Could you check a few things on this model? Use its own coordinates, in mm. Face numbers are marked on the shaded views. Coordinates: 2 decimals unless noted, no trailing zeros. Order: outer loops, then holes, each group sorted by start corner. A loop starts at its lowest first (then second) coordinate and runs counter-clockwise, first axis right, second up. Notation, with made-up numbers: (-31, 48) -> (-6, 48) arc R13 ccw to (-6, 62) -> close; hole circle Ø6 at (65.25, 28.5). An arc over 180 degrees is marked (long way). Use a Markdown table: item, result. Add a question column.
1) Thinking about a two-plate mould opening in Y: for the marked faces 1 and 2, which applies, +Y half, -Y half, draft (parallel to the pull), parting line (faces both ways), or undercut?
2) If we section it at A-A (x = -9): Write out the boundary of the cut face in (y, z) (3 decimals), plus the area to 3 significant figures.
3) If we section it at D-D (x = 1): Write out the boundary of the cut face in (y, z), plus the area to 3 significant figures.
4) Will these pins go through, and if not, where does the flat tip stop? pin 1 Ø3.5 at (x, y) = (18, -18.5) entering from -Z; pin 2 Ø1.1 at (x, y) = (-15.5, -4.5) entering from -Z; pin 3 Ø2.5 at (x, y) = (-9, -18.5) entering from -Z.
5) If we section it at B-B (y = -18.5): Write out the boundary of the cut face in (x, z) (3 decimals).
6) If I drill on L1, parallel to Y at x = 18, z = 2.7 (3 decimals); L2, parallel to Y at x = -9.5, z = 4.65; L3, parallel to X at y = -9.5, z = 0.4, over which ranges is the centre line in solid material (lowest first)? Write a range as [from, to].
7) If we section it at C-C (z = 0.65): Give the number of separate pieces and of enclosed holes in the cut face, plus the area to 3 significant figures.
```python
from build123d import *

# Parameters (mm, degrees)
SKETCH1_W                       = 44
SKETCH1_H                       = 45
BASE_DEPTH                      = 5
WIRE_GROOVES_DEPTH              = 51.338851795
SCREW_INSERTION_HOLE_DEPTH      = 33.181634738
SCREW_INSERTION_HOLE_DEPTH_BACK = 33.181634738
SKETCH3_R                       = 2.75
SKETCH5_W                       = 5
SKETCH5_H                       = 3
ZIP_TIE_SLOTS_DEPTH             = 32.862987933
SKETCH6_R                       = 1.425
MOUNT_CLAMPING_HOLES_DEPTH      = 32.862987933
EDGE_FILLETS_R                  = 1


with BuildPart() as part:
    # Sketch1 → Base (new body)
    with BuildSketch(Plane.XY):
        Rectangle(SKETCH1_W, SKETCH1_H)
    extrude(amount=BASE_DEPTH)

    # Sketch2 → Wire Grooves (cut, through all)
    with BuildSketch(Plane(origin=(0, 22.5, 0), x_dir=(1, 0, 0), z_dir=(0, 1, 0))):
        with BuildLine():
            Line((-18, 0), (-12, 0))
            ThreePointArc((-12, 0), (-12.556497116, -1.343502884), (-13.9, -1.9))
            Line((-13.9, -1.9), (-16.1, -1.9))
            ThreePointArc((-16.1, -1.9), (-17.443502884, -1.343502884), (-18, 0))
        make_face()
        with BuildLine():
            Line((9.9, -1.9), (7.7, -1.9))
            ThreePointArc((7.7, -1.9), (6.356497116, -1.343502884), (5.8, 0))
            Line((5.8, 0), (11.8, 0))
            ThreePointArc((11.8, 0), (11.243502884, -1.343502884), (9.9, -1.9))
        make_face()
    extrude(amount=-WIRE_GROOVES_DEPTH, mode=Mode.SUBTRACT)

    # Sketch3 → Screw Insertion Hole (cut, two sides: drawn at the far end of the back side and taken through both)
    with BuildSketch(Plane(origin=(0, 0.596130014, 4.269237963), x_dir=(-1, 0, 0), z_dir=(0, -0.25881904510252135, -0.9659258262890681)).offset(-SCREW_INSERTION_HOLE_DEPTH_BACK)):
        with Locations(Location((0, 16.291616808, 0), (0, 0, 270))):
            Circle(SKETCH3_R)
    extrude(amount=SCREW_INSERTION_HOLE_DEPTH + SCREW_INSERTION_HOLE_DEPTH_BACK, mode=Mode.SUBTRACT)

    # Sketch5 → Zip Tie Slots (cut, through all)
    with BuildSketch(Plane(origin=(0, 0, 0), x_dir=(-1, 0, 0), z_dir=(0, 0, -1))):
        with Locations((-16, 18)):
            Rectangle(SKETCH5_W, SKETCH5_H)
        with Locations((8, 18)):
            Rectangle(SKETCH5_W, SKETCH5_H)
    extrude(amount=-ZIP_TIE_SLOTS_DEPTH, mode=Mode.SUBTRACT)

    # Sketch6 → Mount Clamping Holes (cut, through all)
    with BuildSketch(Plane(origin=(0, 0, 0), x_dir=(-1, 0, 0), z_dir=(0, 0, -1))):
        with Locations((-18, -18.5)):
            Circle(SKETCH6_R)
        with Locations(Location((9, -18.5, 0), (0, 0, 180))):
            Circle(SKETCH6_R)
    extrude(amount=-MOUNT_CLAMPING_HOLES_DEPTH, mode=Mode.SUBTRACT)

    # Edge Fillets
    edge_fillets_edges = [part.edges().sort_by_distance(p)[0] for p in [
        (-22, 0, 5),
        (0, -22.5, 5),
        (22, 0, 5),
        (22, -22.5, 2.5),
        (-22, -22.5, 2.5),
        (-22, 22.5, 2.5),
        (22, 22.5, 2.5),
        (0, 22.5, 5),
    ]]
    fillet(edge_fillets_edges, radius=EDGE_FILLETS_R)


solid = part.part
```
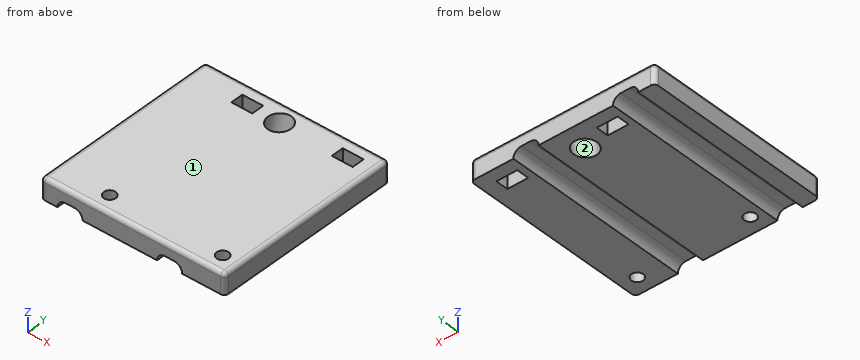
Answer sheet:
| question | item | result |
|---|---|---|
| 1 | face 1 | draft |
| 1 | face 2 | undercut |
| 2 | outline | (-22.5, 0) -> (-19.925, 0) -> (-19.925, 5) -> (-21.5, 5) arc R1 ccw to (-22.5, 4) -> close; (-17.075, 0) -> (16.5, 0) -> (16.5, 5) -> (-17.075, 5) -> close; (19.5, 0) -> (22.5, 0) -> (22.5, 4) arc R1 ccw to (21.5, 5) -> (19.5, 5) -> close |
| 2 | area | 195 mm2 |
| 3 | outline | (-22.5, 0) -> (13.67, 0) -> (15.01, 5) -> (-21.5, 5) arc R1 ccw to (-22.5, 4) -> close; (18.97, 0) -> (22.5, 0) -> (22.5, 4) arc R1 ccw to (21.5, 5) -> (20.31, 5) -> close |
| 3 | area | 198 mm2 |
| 4 | pin 1 | z = 0 |
| 4 | pin 2 | z = 1.9 |
| 4 | pin 3 | through |
| 5 | outline | (-22, 0) -> (-18, 0) arc R1.9 cw to (-16.1, 1.9) -> (-13.9, 1.9) arc R1.9 cw to (-12, 0) -> (-10.425, 0) -> (-10.425, 5) -> (-21, 5) arc R1 ccw to (-22, 4) -> close; (-7.575, 0) -> (5.8, 0) arc R1.9 cw to (7.7, 1.9) -> (9.9, 1.9) arc R1.9 cw to (11.8, 0) -> (16.575, 0) -> (16.575, 5) -> (-7.575, 5) -> close; (19.425, 0) -> (22, 0) -> (22, 4) arc R1 ccw to (21, 5) -> (19.425, 5) -> close |
| 6 | L1 | [-22.5, -19.925], [-17.075, 16.5], [19.5, 22.5] |
| 6 | L2 | [-22.26, -19.83], [-17.17, 16.5], [19.5, 22.26] |
| 6 | L3 | [-22, -17.96], [-12.04, 5.84], [11.76, 22] |
| 7 | separate pieces | 3 |
| 7 | enclosed holes | 5 |
| 7 | area | 1,390 mm2 |
